Check sheet for the modelled part. Datum: model origin and axes. Units: mm. A direction names the side the tool comes from. Give positions to 0.01 mm unless a question says otherwise; leave off trailing zeros. Loops run counter-clockwise (first coordinate to the right, second up) from the corner with the lowest first, then second, coordinate; pieces in that order, holes last. Notation, with made-up numbers: M -31.75,24 L -5.75,24 A23 cw -5.75,49 Z; hole C 66.25,61.25 d2. An arc over 180 degrees is marked long. Use one line per item in the form item = value.
from build123d import *

# Parameters (mm, degrees)
SKETCH1_R             = 7.28
BOSS_EXTRUDE1_DEPTH   = 7.475
CUT_EXTRUDE1_DEPTH    = 8.04
CUT_EXTRUDE2_DEPTH    = 5
CHAMFER2_SIZE         = 0.3
CHAMFER4_SIZE         = 0.3
FILLET1_R             = 0.75
FILLET2_R             = 0.6
FILLET3_R             = 0.3
M3_TAPPED_HOLE3_D     = 2.5
M3_TAPPED_HOLE3_DEPTH = 6
M3_TAPPED_HOLE3_TIP   = 0.751075774
M3_TAPPED_HOLE4_D     = 2.5
M3_TAPPED_HOLE4_DEPTH = 6.5
M3_TAPPED_HOLE4_TIP   = 0.751075774


with BuildPart() as part:
    # Sketch1 → Boss-Extrude1 (new, symmetric)
    with BuildSketch(Plane.XY):
        Circle(SKETCH1_R)
    extrude(amount=BOSS_EXTRUDE1_DEPTH, both=True)

    # Sketch3 → Cut-Extrude1 (cut)
    with BuildSketch(Plane.XY.offset(7.475)):
        with BuildLine():
            Line((2, 4.341474404), (2, -4.341474404))
            ThreePointArc((2, -4.341474404), (0, -4.78), (-2, -4.341474404))
            Line((-2, -4.341474404), (-2, 4.341474404))
            ThreePointArc((-2, 4.341474404), (0, 4.78), (2, 4.341474404))
        make_face()
    extrude(amount=-CUT_EXTRUDE1_DEPTH, mode=Mode.SUBTRACT)

    # Sketch4 → Cut-Extrude2 (cut)
    with BuildSketch(Plane(origin=(0, 0, -7.475), x_dir=(-1, 0, 0), z_dir=(0, 0, -1))):
        with BuildLine():
            Line((-1.5, 1.974943037), (-1.5, -1.974943037))
            ThreePointArc((-1.5, -1.974943037), (0, -2.48), (1.5, -1.974943037))
            Line((1.5, -1.974943037), (1.5, 1.974943037))
            ThreePointArc((1.5, 1.974943037), (0, 2.48), (-1.5, 1.974943037))
        make_face()
    extrude(amount=-CUT_EXTRUDE2_DEPTH, mode=Mode.SUBTRACT)

    # Chamfer2
    chamfer2_edges = [part.edges().sort_by_distance(p)[0] for p in [
        (1.5, 0, -2.475),
        (-1.5, 0, -2.475),
    ]]
    chamfer(chamfer2_edges, length=CHAMFER2_SIZE)

    # Chamfer4
    chamfer4_edges = [part.edges().sort_by_distance(p)[0] for p in [
        (0, 2.48, -7.475),
        (-1.5, 0, -7.475),
        (0, -2.48, -7.475),
        (1.5, 0, -7.475),
    ]]
    chamfer(chamfer4_edges, length=CHAMFER4_SIZE)

    # Fillet1
    fillet1_edges = [part.edges().sort_by_distance(p)[0] for p in [
        (-7.28, 0, -7.475),
        (-7.28, 0, 7.475),
    ]]
    fillet(fillet1_edges, radius=FILLET1_R)

    # Fillet2
    fillet2_edges = [part.edges().sort_by_distance(p)[0] for p in [
        (0, -4.78, -0.565),
        (0, 4.78, -0.565),
    ]]
    fillet(fillet2_edges, radius=FILLET2_R)

    # Fillet3
    fillet3_edges = [part.edges().sort_by_distance(p)[0] for p in [
        (0, 2.48, -2.475),
        (0, -2.48, -2.475),
    ]]
    fillet(fillet3_edges, radius=FILLET3_R)

    # M3 Tapped Hole3
    with Locations(Plane(origin=(7.28, 0, 0), x_dir=(0, 0, -1), z_dir=(1, 0, 0))):
        with Locations((-3.3625, 0)):
            Hole(M3_TAPPED_HOLE3_D / 2, depth=M3_TAPPED_HOLE3_DEPTH)
            with Locations((0, 0, -(M3_TAPPED_HOLE3_DEPTH + M3_TAPPED_HOLE3_TIP / 2))):  # 118° drill point
                Cone(0, M3_TAPPED_HOLE3_D / 2, M3_TAPPED_HOLE3_TIP, mode=Mode.SUBTRACT)

    # M3 Tapped Hole4
    with Locations(Plane(origin=(7.28, 0, 0), x_dir=(0, 0, -1), z_dir=(1, 0, 0))):
        with Locations((4.41685425, 0)):
            Hole(M3_TAPPED_HOLE4_D / 2, depth=M3_TAPPED_HOLE4_DEPTH)
            with Locations((0, 0, -(M3_TAPPED_HOLE4_DEPTH + M3_TAPPED_HOLE4_TIP / 2))):  # 118° drill point
                Cone(0, M3_TAPPED_HOLE4_D / 2, M3_TAPPED_HOLE4_TIP, mode=Mode.SUBTRACT)


solid = part.part
1) Section check A-A (y = 0). State how many separate pieces and enclosed holes the cut face has, then the cut area to 3 significant figures.
Evaluation:
separate_pieces = 3
enclosed_holes = 0
area = 142 mm^2
2) Section check B-B (x = 0). Record the cut outline in (y, z) (3 decimals), then the cut area to 3 significant figures.
Evaluation:
outline = M -7.28,-6.725 A0.75 ccw -6.53,-7.475 L -2.78,-7.475 L -2.48,-7.175 L -2.48,-2.775 A0.3 cw -2.18,-2.475 L 2.18,-2.475 A0.3 cw 2.48,-2.775 L 2.48,-7.175 L 2.78,-7.475 L 6.53,-7.475 A0.75 ccw 7.28,-6.725 L 7.28,6.725 A0.75 ccw 6.53,7.475 L 4.78,7.475 L 4.78,0.035 A0.6 cw 4.18,-0.565 L -4.18,-0.565 A0.6 cw -4.78,0.035 L -4.78,7.475 L -6.53,7.475 A0.75 ccw -7.28,6.725 Z
area = 116 mm^2
3) Section check D-D (z = -3.5). Record the cut outline in (x, y).
Evaluation:
outline = M -1.5,-1.97 L -1.5,1.97 A2.48 cw 1.5,1.97 L 1.5,0.85 L 7.23,0.85 A7.28 ccw long 7.23,-0.85 L 1.5,-0.85 L 1.5,-1.97 A2.48 cw Z
4) Set-up check for faces 1 (the face through (-2, 0, 4)), 2 (the face through (4.35, 0.375, -3.225)), 3 (the face through (3, 0, 7.475)), 4 (the face through (0, 0, -2.475)), 5 (the face through (3, 0, -7.475)): record each of +Z, -Z, +X, -X, +Y, -Y from which the full face is reachable in a straight line by a thin tool's end or side.
Evaluation:
face_1 = +Z
face_2 = +X
face_3 = +Z, +X, -X, +Y, -Y
face_4 = -Z
face_5 = -Z, +X, -X, +Y, -Y
5) Depth check by flat-ended pin: pin 1 Ø2.5 at (x, y) = (0.5, -0.5) entering from -Z (3 decimals); pin 2 Ø2 at (y, z) = (-2, 5) entering from +X; pin 3 Ø1.2 at (x, y) = (0.5, 0) entering from +Z (3 decimals). Enter the tip coordinate at first touch or a pass-through.
Evaluation:
pin_1 = -7.425
pin_2 = 7.21
pin_3 = -0.565
6) Section check C-C (z = 2.75). Record the cut outline in (x, y).
Evaluation:
outline = M -2,-4.34 L -2,4.34 A4.78 cw 2,4.34 L 2,1.09 L 7.2,1.09 A7.28 ccw long 7.2,-1.09 L 2,-1.09 L 2,-4.34 A4.78 cw Z
7) Scan lines: line 1 (Z direction, x = 6, y = 0) (1 decimal); line 2 (X direction, y = 0.25, z = -0.25); line 3 (Z direction, x = 3.5, y = 0.25) (3 decimals). Record each from-to range of solid material in increasing order.
Evaluation:
line_1 = -7.5 to -5.7, -3.2 to 2.1, 4.6 to 7.5
line_2 = -7.28 to -2, 2 to 7.28
line_3 = -7.475 to -5.642, -3.192 to 2.138, 4.587 to 7.475
8) Release check for a two-part mould opening along X. For faces 6 (the face through (-2, -7, 0)), 7 (the face through (4.603, 0.055, 2.114)), 8 (the face through (0.03, -4.78, 3.81)) record: pulls with the +X half, pulls with the -X half, needs draft (parallel to the pull), parting line crosses it, or undercut.
Evaluation:
face_6 = parting line crosses it
face_7 = needs draft
face_8 = undercut
